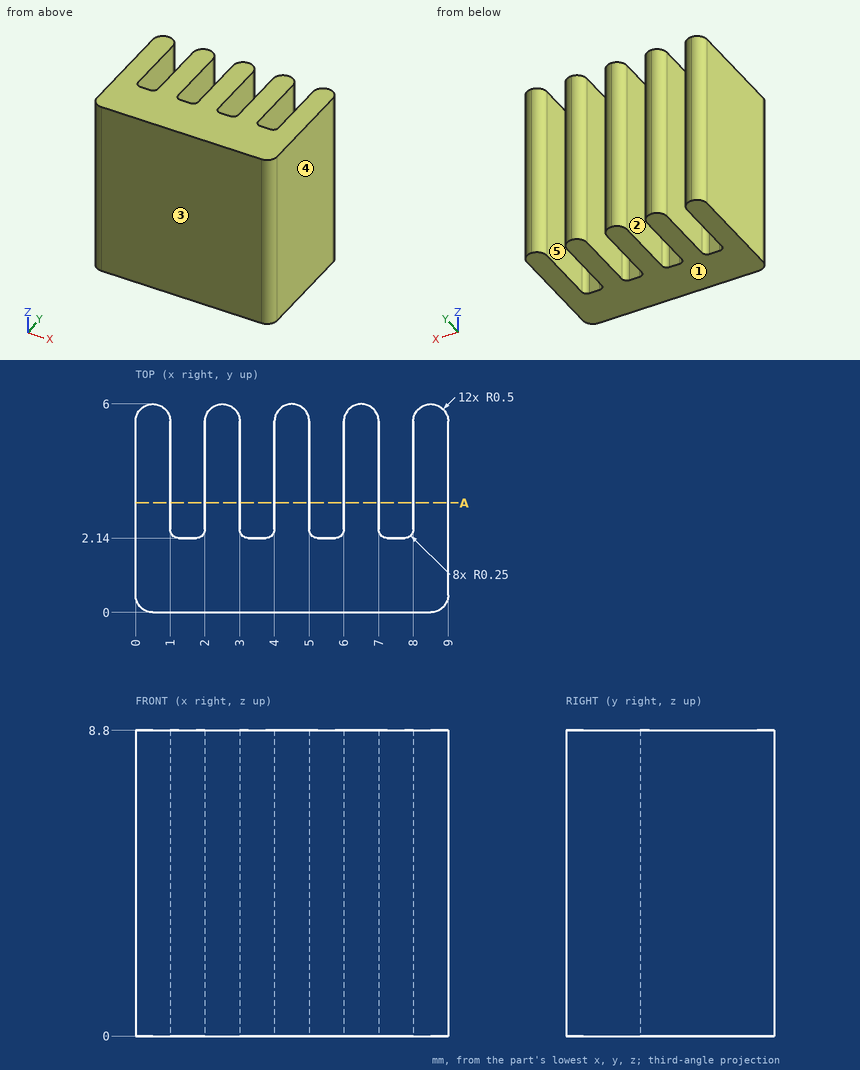
Input: dimensioned drawing with shaded views. Units: mm. Origin: part minimum x, y, z. A direction names the side the tool comes from. Coordinates: 2 decimals unless noted, no trailing zeros. Order: outer loops, then holes, each group sorted by start corner. A loop starts at its lowest first (then second) coordinate and runs counter-clockwise, first axis right, second up. Notation, with made-up numbers: M 57,41 L 80,41 A13 cw 80,57 Z; hole C 57.5,45 d6. An arc over 180 degrees is marked long. Answer as CSV lines item,"result".
Q1. Draft query along X for the marked faces 3, 4 and 5. Return one class per face: pulls with the +X half, pulls with the -X half, needs draft (parallel to the pull), parting line crosses it, or undercut.
Answers:
face 3,"needs draft"
face 4,"pulls with the +X half"
face 5,"undercut"
Q2. Set-up query: the marked faces 1 and 2. Return all of +Z, -Z, +X, -X, +Y, -Y with unobstructed straight access to the full face (end or side cutting, diameter ignored); none if empty.
Answers:
face 1,"-Z, +X, -X, +Y, -Y"
face 2,"+Z, -Z, +Y"
Q3. Section A-A on y = 3.15. Return the cut outline in (x, z), and give its area (3 significant figures).
Answers:
outline,"M 0,0 L 1,0 L 1,8.8 L 0,8.8 Z; M 2,0 L 3,0 L 3,8.8 L 2,8.8 Z; M 4,0 L 5,0 L 5,8.8 L 4,8.8 Z; M 6,0 L 7,0 L 7,8.8 L 6,8.8 Z; M 8,0 L 9,0 L 9,8.8 L 8,8.8 Z"
area,"44.0 mm^2"
Q4. First-contact query: P1, Ø0.6, axis at x = 5.5, z = 6.5, coming from the +Y side (3 decimals). Flat tip, straight axial feed; report the tip coordinate or a pass-through.
Answers:
P1,"stops at y = 2.145"
Q5. Line query: probe 1 along X at (y, z) = (2.6, 6.25); probe 2 along Y at (x, z) = (5.75, 5.5); probe 3 along Y at (x, z) = (2.25, 7). Output: solid intervals per line, ascending. Write a range as [from, to].
Answers:
probe 1,"x = [0, 1], [2, 3], [4, 5], [6, 7], [8, 9]"
probe 2,"y = [0, 2.14]"
probe 3,"y = [0, 5.93]"
